Input: part model. Units: mm. Frame: model coordinates. Round coordinates to 2 decimals unless told otherwise and drop trailing zeros. Loops run counter-clockwise (first coordinate to the right, second up) from the corner with the lowest first, then second, coordinate; pieces in that order, holes last. Notation, with made-up numbers: (-25.75, -38.5) -> (-12.75, -38.5) arc R19 cw to (-12.75, -13.5) -> close; hole circle Ø11 at (-19.75, 89). An arc over 180 degrees is marked (long way). One line per question, with ' | ' between items. Start each with the question number.
Q1. Cut plane A-A on x = 18. Return loops of the section in (y, z).
Q2. Cut plane D-D on z = 17. Return loops of the section in (x, y).
Q3. Contact query for a flat-ended pin moving along its axis: P1, Ø6, axis at x = 14, y = -0.5, coming from the -Z side. Output: stop coordinate, or through.
Q4. Material intervals for L1, parallel to X at y = 0, z = 33; L2, parallel to Y at x = 10.5, z = 74; L3, parallel to X at y = 1, z = 80, sorted ascending.
Q5. Cut plane B-B on y = 0. Return loops of the section in (x, z).
Q6. Cut plane C-C on z = 43.5. Return loops of the section in (x, y), and give its area (3 significant figures).
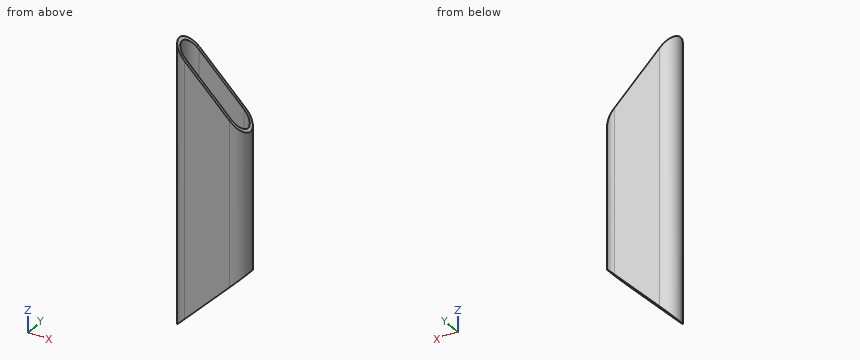
from build123d import *

# Parameters (mm, degrees)
BOSS_EXTRUDE1_DEPTH = 130
CUT_EXTRUDE1_DEPTH  = 30


with BuildPart() as part:
    # Sketch1 → Boss-Extrude1 (new body)
    with BuildSketch(Plane.XY):
        with BuildLine():
            Line((0, 6), (21, 6))
            ThreePointArc((21, 6), (27, 0), (21, -6))
            Line((21, -6), (0, -6))
            ThreePointArc((0, -6), (-6, 0), (0, 6))
        make_face()
        with BuildLine():
            Line((0, 4.8), (21, 4.8))
            ThreePointArc((21, 4.8), (25.8, 0), (21, -4.8))
            Line((21, -4.8), (0, -4.8))
            ThreePointArc((0, -4.8), (-4.8, 0), (0, 4.8))
        make_face(mode=Mode.SUBTRACT)
    extrude(amount=BOSS_EXTRUDE1_DEPTH)

    # Sketch2 → Cut-Extrude1 (cut)
    with BuildSketch(Plane(origin=(0, 6, 0), x_dir=(1, 0, 0), z_dir=(0, 1, 0))):
        Polygon((-6, 0), (27, -33), (27, 0), align=None)
        Polygon((-6, -130), (27, -97), (27, -130), align=None)
    extrude(amount=-CUT_EXTRUDE1_DEPTH, mode=Mode.SUBTRACT)


solid = part.part
Results:
1) outline: (-6, 24) -> (-4.8, 24) -> (-4.8, 106) -> (-6, 106) -> close; (4.8, 24) -> (6, 24) -> (6, 106) -> (4.8, 106) -> close
2) outline: (0, -6) -> (11, -6) -> (11, -4.8) -> (0, -4.8) arc R4.8 cw to (0, 4.8) -> (11, 4.8) -> (11, 6) -> (0, 6) arc R6 ccw to start
3) P1: through
4) L1: -6 to -4.8, 25.8 to 27 | L2: -6 to -4.8, 4.8 to 6 | L3: -5.92 to -4.69, 25.69 to 26.92
5) outline: (-6, 0) -> (-4.8, 1.2) -> (-4.8, 128.8) -> (-6, 130) -> close; (25.8, 31.8) -> (27, 33) -> (27, 97) -> (25.8, 98.2) -> close
6) outline: (0, -6) -> (21, -6) arc R6 ccw to (21, 6) -> (0, 6) arc R6 ccw to start; hole (0, -4.8) -> (21, -4.8) arc R4.8 ccw to (21, 4.8) -> (0, 4.8) arc R4.8 ccw to start | area: 91.1 mm^2
